The listing builds one solid part. Answer for the finished solid, in the listing's coordinates (mm). Face numbers are marked on the shaded views. A direction names the side the tool comes from. Round coordinates to 2 decimals unless told otherwise and drop trailing zeros. Write each loop counter-clockwise with the first axis right and the second up, starting at its lowest first coordinate (ties: lowest second). Pieces come first, ordered by that corner, then holes. Notation, with made-up numbers: M 62.5,60.25 L 118.5,60.25 A24 ccw 118.5,96.25 Z; hole C -23.75,-6.75 d10. An arc over 180 degrees is marked long. Put each result on its own line as item: value. Start each with the question number.
```python
from build123d import *

# Parameters (mm, degrees)
F1_DEPTH = 5
F2_SIZE  = 20
F3_R     = 9.99999


# Not quite as in the source:
# - a fillet or chamfer is up to 0.001 mm smaller than in the source, because OpenCascade refuses the exact size
# - a feature names something its author has since deleted; it is built from what else it names


with BuildPart() as f1:
    # F0 (on Top) → F1 (new body)
    with BuildSketch(Plane.XY):
        Polygon((0, -28.6713610368), (0, -25.9807621135), (-11.250000041, -19.4855715615), (-22.5, -12.9903810568), (-22.5, 0), (-22.5, 11.8356805184), (-32.5, 11.8356805184), (-32.5, -43.6713610368), (0, -43.6713610368), (0, -38.6713610368), (-5, -38.6713610368), (-5, -28.6713610368), align=None)
        Polygon((11.2499998166, -19.485571691), (0, -25.9807621135), (0, -28.6713610368), (5, -28.6713610368), (5, -38.6713610368), (0, -38.6713610368), (0, -43.6713610368), (32.5, -43.6713610368), (32.5, 11.8356805184), (22.5, 11.8356805184), (22.5, 0), (22.5, -12.9903810568), align=None)
    extrude(amount=F1_DEPTH)

    # F2
    f2_edges = [f1.edges().sort_by_distance(p)[0] for p in [
        (-32.5, -43.671361, 2.5),
        (32.5, -43.671361, 2.5),
    ]]
    chamfer(f2_edges, length=F2_SIZE)

    # F3 (radius 10 in the source; OpenCascade refuses exactly that, so slightly less here)
    f3_edges = [f1.edges().sort_by_distance(p)[0] for p in [
        (-32.5, 11.835681, 2.5),
        (32.5, -23.671361, 2.5),
        (32.5, 11.835681, 2.5),
        (12.5, -43.671361, 2.5),
        (-12.5, -43.671361, 2.5),
        (-32.5, -23.671361, 2.5),
    ]]
    fillet(f3_edges, radius=F3_R)


solid = f1.part
```
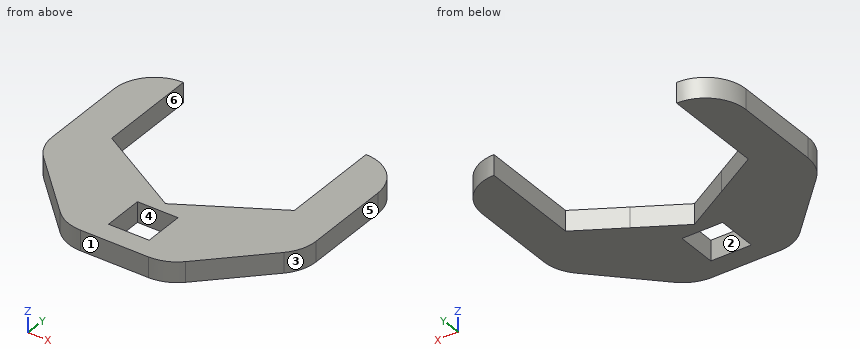
Item 1: Determine the mould class of the marked faces 1, 2 and 3 for opening direction X: released by +X, released by -X, zero draft, split by the parting line, or undercut.
Item 2: Which of the six approach directions +Z, -Z, +X, -X, +Y, -Y give full straight-line access (tool end or side, diameter ignored) to the marked faces 4, 5 and 6?
Item 3: Consider line 1 along X through (y, z) = (-7.5, 0.85); line 2 along Y through (x, z) = (-3, 1.6); line 3 along X through (y, z) = (-18.5, 1.9). Determine where each line is inside the solid, lowest interval first. Write a range as [from, to].
Item 4: Section A-A (y = -7.5) is taken. Give the vertices of the cut face in (x, z), and give its area (3 significant figures).
Item 5: Section D-D (y = -40) is taken. Give the vertices of the cut face in (x, z).
Item 6: Section C-C (x = -23.5) is taken. Give the vertices of the cut face in (y, z).
Item 7: Flat-ended cylindrical pins translate along their axes: pin 1 (6 mm diameter, centred on x = 19, y = -8.5, fed in from +Z); pin 2 (3 mm diameter, centred on y = -23, z = 3.5, fed in from -X); pin 3 (1.5 mm diameter, centred on y = -32.5, z = 2, fed in from -X). Find the tip coordinate at first contact, or state that the pin passes through.
Output values:
1. face 1: zero draft
1. face 2: undercut
1. face 3: released by +X
2. face 4: +Z, -Z
2. face 5: +Z, -Z, +X, +Y, -Y
2. face 6: +Z, -Z, +Y
3. line 1: x = [-32.5, -22.5], [22.5, 32.5]
3. line 2: y = [-43.67, -38.67], [-28.67, -24.25]
3. line 3: x = [-32.5, -12.96], [12.96, 32.5]
4. outline: M -32.5,0 L -22.5,0 L -22.5,5 L -32.5,5 Z; M 22.5,0 L 32.5,0 L 32.5,5 L 22.5,5 Z
4. area: 100 mm^2
5. outline: M -16.17,0 L 16.17,0 L 16.17,5 L -16.17,5 Z
6. outline: M -32.67,0 L 11.79,0 L 11.79,5 L -32.67,5 Z
7. pin 1: passes through
7. pin 2: stops at x = -32.3
7. pin 3: stops at x = -24.42
